Autodesk Inventor part; units mm, degrees
ref_plane "YZ Plane" through (0, 0, 0) normal (1, 0, 0) x (0, 1, 0)
ref_plane "XZ Plane" through (0, 0, 0) normal (0, 1, 0) x (-1, 0, 0)
ref_plane "XY Plane" through (0, 0, 0) normal (0, 0, 1) x (1, 0, 0)
sketch "Sketch1" plane through (0, 0, 0) normal (0, 1, 0) x (-1, 0, 0)
  circle A0 centre (-27.7235, -39.6791) radius 2.3
  line L0 (24.7765, 36.3209) -> (-27.7235, -39.6791)
  circle A1 centre (24.7765, -39.6791) radius 2.3
  circle A2 centre (-27.7235, 36.3209) radius 2.3
  line L1 (24.7765, -39.6791) -> (-27.7235, 36.3209)
  circle A3 centre (24.7765, 36.3209) radius 2.3
  circle A4 centre (24.7765, 36.3209) radius 2.3
  circle A5 centre (-27.7235, 36.3209) radius 2.3
  circle A6 centre (24.7765, -39.6791) radius 2.3
  circle A7 centre (-27.7235, -39.6791) radius 2.3
  circle A8 centre (-1.4735, -1.6791) radius 6.8323
  circle A9 centre (-27.7235, 36.3209) radius 5
  circle A10 centre (-27.7235, -39.6791) radius 5
  circle A11 centre (24.7765, -39.6791) radius 5
  circle A12 centre (24.7765, 36.3209) radius 5
  line L2 (-27.7235, 41.3209) -> (-18.7235, 41.3209)
  line L3 (-18.7235, 41.3209) -> (-18.7235, 31.3209)
  line L4 (-18.7235, 31.3209) -> (-27.7235, 31.3209)
  line L5 (24.7765, 41.3209) -> (15.7765, 41.3209)
  line L6 (15.7765, 41.3209) -> (15.7765, 31.3209)
  line L7 (15.7765, 31.3209) -> (24.7765, 31.3209)
  line L8 (24.7765, -34.6791) -> (15.7765, -34.6791)
  line L9 (15.7765, -34.6791) -> (15.7765, -44.6791)
  line L10 (15.7765, -44.6791) -> (24.7765, -44.6791)
  line L11 (-27.7235, -34.6791) -> (-18.7235, -34.6791)
  line L12 (-18.7235, -34.6791) -> (-18.7235, -44.6791)
  line L13 (-18.7235, -44.6791) -> (-27.7235, -44.6791)
  point P0 (0, 0)
  dimension "d0" = 10
  dimension "d1" = 10
  dimension "d2" = 10
  dimension "d3" = 10
  dimension "d4" = 9
  dimension "d5" = 9
extrude "Extrusion1" add sketch "Sketch1" along normal blind 10 contours A10 | A10 L11 L0 | L0 L11 L12 L13 A10 | L4 A9 L1 | L1 A9 L2 L3 L4 | L7 L6 L5 A12 L0 | L0 A12 L7 | L8 A11 L1 | L1 A11 L10 L9 L8 | A9 | A11 | A12
sketch "Sketch2" plane through (0, 10, 0) normal (0, 1, 0) x (1, 0, 0)
  line L0 (-15.7765, -41.3209) -> (-15.7765, -31.3209)
  line L1 (-15.7765, -31.3209) -> (-24.7765, -31.3209)
  line L2 (-15.7765, -41.3209) -> (-20.2765, -41.3209)
  line L3 (-20.2765, -41.3209) -> (-20.2765, -31.3209)
  line L4 (-20.2765, -31.3209) -> (-15.7765, -31.3209)
  line L5 (-15.7765, -31.3209) -> (-15.7765, -41.3209)
  line L6 (-24.7765, 34.6791) -> (-15.7765, 34.6791)
  line L7 (-15.7765, 44.6791) -> (-24.7765, 44.6791)
  line L8 (-15.7765, 34.6791) -> (-20.2765, 34.6791)
  line L9 (-20.2765, 34.6791) -> (-20.2765, 44.6791)
  line L10 (-20.2765, 44.6791) -> (-15.7765, 44.6791)
  line L11 (-15.7765, 44.6791) -> (-15.7765, 34.6791)
  line L12 (18.7235, 34.6791) -> (23.2235, 34.6791)
  line L13 (23.2235, 34.6791) -> (23.2235, 44.6791)
  line L14 (23.2235, 44.6791) -> (18.7235, 44.6791)
  line L15 (18.7235, 44.6791) -> (18.7235, 34.6791)
  line L16 (18.7235, -41.3209) -> (27.7235, -41.3209)
  line L17 (18.7235, -41.3209) -> (23.2235, -41.3209)
  line L18 (23.2235, -41.3209) -> (23.2235, -31.3209)
  line L19 (23.2235, -31.3209) -> (18.7235, -31.3209)
  line L20 (18.7235, -31.3209) -> (18.7235, -41.3209)
  point P0 (0, 0)
extrude "Extrusion2" add sketch "Sketch2" along normal blind 45
sketch "Sketch3" plane through (0, 55, 0) normal (0, 1, 0) x (1, 0, 0)
  line L0 (-20.2765, -41.3209) -> (-20.2765, -31.3209)
  line L1 (27.7235, 44.6791) -> (18.7235, 44.6791)
  line L2 (-20.2765, -41.3209) -> (23.2235, -41.3209)
  line L3 (23.2235, -41.3209) -> (23.2235, 44.6791)
  line L4 (23.2235, 44.6791) -> (-20.2765, 44.6791)
  line L5 (-20.2765, 44.6791) -> (-20.2765, -41.3209)
  point P0 (0, 0)
extrude "Extrusion3" add sketch "Sketch3" along normal blind 8
sketch "Sketch4" plane through (0, 63, 0) normal (0, 1, 0) x (1, 0, 0)
  line L0 (-20.2765, 44.6791) -> (-20.2765, -41.3209)
  line L1 (-20.2765, -41.3209) -> (23.4801, 44.6791)
  line L2 (23.2235, -41.3209) -> (23.2235, 44.6791)
  line L3 (23.2235, 44.6791) -> (-20.2765, 44.6791)
  line L4 (23.2235, -41.3209) -> (-20.2765, 44.6791)
  circle A0 centre (1.4735, 1.6791) radius 6.5
  line L5 (17.4735, 5.6791) -> (-14.5265, 5.6791)
  line L6 (-14.5265, 5.6791) -> (-14.5265, -2.3209)
  line L7 (-14.5265, -2.3209) -> (17.4735, -2.3209)
  line L8 (17.4735, -2.3209) -> (17.4735, 5.6791)
  line L9 (17.4735, 5.6791) -> (-14.5265, -2.3209) construction
  line L10 (-14.5265, 5.6791) -> (17.4735, -2.3209) construction
  point P0 (0, 0)
  point P1 (-3.65, 5.6791)
  point P2 (-3.65, -2.3209)
  point P3 (6.597, -2.3209)
  point P4 (6.597, 5.6791)
  dimension "d13" = 13
  dimension "d14" = 32
  dimension "d15" = 8
extrude "Extrusion4" cut sketch "Sketch4" against normal blind 5 contours A0 L1 L5 L4 | L4 L5 A0 | A0 L7 L1 | L1 L7 L4 A0 | L5 L1 L4 | L4 L1 L7 A0 L5 | A0 L5 L1 | A0 L7 L6 L5 | L1 L4 L7 | L4 L7 A0 | L1 L5 A0 L7 L4 | L5 L8 L7 A0
sketch "Sketch5" plane through (0, 58, 0) normal (0, 1, 0) x (1, 0, 0)
  arc A0 (6.597, 5.6791) -> (-3.65, 5.6791) centre (1.4735, 1.6791) ccw
  arc A1 (-3.65, -2.3209) -> (6.597, -2.3209) centre (1.4735, 1.6791) ccw
  circle A2 centre (1.4735, 1.6791) radius 2.25
  point P0 (0, 0)
  dimension "d18" = 4.5
extrude "Extrusion5" cut sketch "Sketch5" against normal blind 8
properties part number "ATTACHMENT_TOOLHEAD_GRIPPER"
Design review of the part built by this model. Coordinates are the model's own, in mm. A direction names the side the tool comes from. Give positions to 0.01 mm unless a question says otherwise; leave off trailing zeros. Loops run counter-clockwise (first coordinate to the right, second up) from the corner with the lowest first, then second, coordinate; pieces in that order, holes last. Notation, with made-up numbers: M 66,61 L 85,61 A13 ccw 85,81 Z; hole C 2.25,30.5 d11. An arc over 180 degrees is marked long. One line per question, with ' | ' between items. Start each with the question number.
1. Add section D-D (y = 8). Write out the cut boundary in (x, z), plus the area to 3 significant figures.
2. For faces 4 (the face through (1.56, 60.54, -8.18)), 5 (the face through (-15.776, 27, 36)), 6 (the face through (-19, 21, 31.321)), 7 (the face through (29.42, 4.93, 34.77)), 8 (the face through (-21, 0, -40)), list the 3-axis set-ups (+Z, -Z, +X, -X, +Y, -Y) from which the entire face can be reached by the end or side of a thin tool; tool diameter is ignored.
3. Add section A-A (y = 36.5). Write out the cut boundary in (x, z), plus the area to 3 significant figures.
4. Add section C-C (x = 0.5). Write out the cut boundary in (y, z), plus the area to 3 significant figures.
5. The part is to be moulded in two halves that separate along X. For faces 1 (the face through (-24, 10, -37)), 2 (the face through (6, 55, -2)), 3 (the face through (-20.276, 56, -8)), say which applies: released by +X, released by -X, zero draft, split by the parting line, or undercut.
6. Insertion check: P1, Ø5, axis at x = 28.5, z = -39, coming from the +Y side; P2, Ø5, axis at y = 31.5, z = -40, coming from the +X side; P3, Ø1, axis at x = 11, z = -28.5, coming from the -Y side; P4, Ø5.5, axis at x = -24.78, z = 36.32, coming from the -Y side. Each pin has a flat end and moves straight along its axis. Give the tip position at first contact, or say it passes through.
7. Add section B-B (x = -7.5). Write out the cut boundary in (y, z), plus the area to 3 significant figures.
8. To check wall thickness, follow L1, parallel to Y at x = -20, z = 18; L2, parallel to X at y = 42, z = 32; L3, parallel to Z at x = -19, y = 33.5. State the ranges of each line that lie inside material, in increasing order.
Worked out:
1) outline: M -24.78,-44.68 L -15.78,-44.68 L -15.78,-34.68 L -24.78,-34.68 A5 ccw Z; M -24.78,31.32 L -15.78,31.32 L -15.78,41.32 L -24.78,41.32 A5 ccw Z; M 18.72,-44.68 L 27.72,-44.68 A5 ccw 27.72,-34.68 L 18.72,-34.68 Z; M 18.72,31.32 L 27.72,31.32 A5 ccw 27.72,41.32 L 18.72,41.32 Z; hole C -24.78,-39.68 d4.6; hole C -24.78,36.32 d4.6; hole C 27.72,-39.68 d4.6; hole C 27.72,36.32 d4.6 | area: 451 mm²
2) face 4: +Y | face 5: +Z, -Z, -Y | face 6: +X, -X, -Y | face 7: +Y, -Y | face 8: +Z, -Z, +X, -X, -Y
3) outline: M -20.28,-44.68 L -15.78,-44.68 L -15.78,-34.68 L -20.28,-34.68 Z; M -20.28,31.32 L -15.78,31.32 L -15.78,41.32 L -20.28,41.32 Z; M 18.72,-44.68 L 23.22,-44.68 L 23.22,-34.68 L 18.72,-34.68 Z; M 18.72,31.32 L 23.22,31.32 L 23.22,41.32 L 18.72,41.32 Z | area: 180 mm²
4) outline: M 55,-44.68 L 63,-44.68 L 63,-8.11 L 58,-8.11 L 58,-3.71 L 55,-3.71 Z; M 55,0.35 L 58,0.35 L 58,4.75 L 63,4.75 L 63,41.32 L 55,41.32 Z | area: 612 mm²
5) face 1: zero draft | face 2: undercut | face 3: released by -X
6) P1: stops at y = 10 | P2: stops at x = 23.22 | P3: stops at y = 55 | P4: stops at y = 0
7) outline: M 55,-44.68 L 63,-44.68 L 63,-5.68 L 58,-5.68 L 58,2.32 L 63,2.32 L 63,41.32 L 55,41.32 Z | area: 648 mm²
8) L1: y = 55 to 63 | L2: x = -20.28 to -15.78, 18.72 to 23.22 | L3: z = -44.68 to -34.68, 31.32 to 41.32
